Geometry: final body of the model. Coordinates: model frame, mm. A direction names the side the tool comes from. Give positions to 0.01 mm unless a question says otherwise; leave off trailing zeros. Loops run counter-clockwise (first coordinate to the right, second up) from the corner with the lowest first, then second, coordinate; pieces in that order, holes last.
from build123d import *

# Parameters (mm, degrees)
F1_DEPTH = 11.34999
F2_R     = 5.674985
F3_R     = 2.5
F4_DEPTH = 24.53132
F5_R     = 3.69316
F6_R     = 1.98374
F7_R     = 1.35255
F8_DEPTH = 1.70942


# Not quite as in the source:
# - a fillet or chamfer is up to 0.001 mm smaller than in the source, because OpenCascade refuses the exact size


with BuildPart() as f1:
    # F0 (on Top) → F1 (new body)
    with BuildSketch(Plane.XY):
        Polygon((-20.0249917, 0), (0, 0), (0, -21.11248), (-20.0249917, -21.11248), (-20.0249917, -22.8219), (1.70942, -22.8219), (1.70942, 1.70942), (-20.0249917, 1.70942), align=None)
    extrude(amount=F1_DEPTH)

    # F2 (radius 5.674995 in the source; OpenCascade refuses exactly that, so slightly less here)
    f2_edges = [f1.edges().sort_by_distance(p)[0] for p in [
        (-20.024992, -21.96719, 11.34999),
        (-20.024992, -21.96719, 0),
        (-20.024992, 0.85471, 11.34999),
        (-20.024992, 0.85471, 0),
    ]]
    fillet(f2_edges, radius=F2_R)

    # F3 (on face) → F4 (cut, through all)
    with BuildSketch(Plane.XZ.offset(22.8219)):
        with Locations((-14.3499967, 5.674995)):
            Circle(F3_R)
    extrude(amount=-F4_DEPTH, mode=Mode.SUBTRACT)

    # F5
    f5_edges = [f1.edges().sort_by_distance(p)[0] for p in [
        (1.70942, -22.8219, 5.674995),
        (1.70942, 1.70942, 5.674995),
    ]]
    fillet(f5_edges, radius=F5_R)

    # F6
    f6_edges = [f1.edges().sort_by_distance(p)[0] for p in [
        (0, -21.11248, 5.674995),
        (0, 0, 5.674995),
    ]]
    fillet(f6_edges, radius=F6_R)

    # F7 (on face) → F8 (cut, through all)
    with BuildSketch(Plane(origin=(0, 0, 0), x_dir=(0, -1, 0), z_dir=(-1, 0, 0))):
        with Locations((15.95374, 5.674995)):
            Circle(F7_R)
        with Locations((5.15874, 5.674995)):
            Circle(F7_R)
    extrude(amount=-F8_DEPTH, mode=Mode.SUBTRACT)


solid = f1.part
Item 1: Section query A-A on x = -8.5. Return loops of the section in (y, z).
Values follow:
outline: (-22.82, 0) - (-21.11, 0) - (-21.11, 11.35) - (-22.82, 11.35) - close; (0, 0) - (1.71, 0) - (1.71, 11.35) - (0, 11.35) - close
Item 2: Set-up query: faces 5 (the face through (-11, -21.112, 6)), 6 (the face through (1.709, -11, 6)). Return all of +Z, -Z, +X, -X, +Y, -Y with unobstructed straight access to the full face (end or side cutting, diameter ignored); none if empty.
Values follow:
face 5: +Z, -Z, -X
face 6: +Z, -Z, +X, +Y, -Y
Item 3: Section query D-D on y = -15.25. Return loops of the section in (x, z).
Values follow:
outline: (0, 0) - (1.71, 0) - (1.71, 4.52) - (0, 4.52) - close; (0, 6.83) - (1.71, 6.83) - (1.71, 11.35) - (0, 11.35) - close
Item 4: Pin query (flat end, axial travel): pin 1 (3.5 mm diameter, centred on y = -5.16, z = 5.67, fed in from +X); pin 2 (2 mm diameter, centred on y = -13.5, z = 5, fed in from -X). Return the tip coordinate at first contact, or that it passes through.
Values follow:
pin 1: stops at x = 1.71
pin 2: stops at x = 0
Item 5: Draft query along Z for faces 1 (the face through (-0.597, -0.566, 5.754)), 2 (the face through (-18.41, 0.84, 9.64)), 3 (the face through (-18.4, 0.8, 1.7)), 4 (the face through (-14.675, -21.979, 8.154)). Return one class per face: +Z half, -Z half, draft (parallel to the pull), parting line (faces both ways), or undercut.
Values follow:
face 1: draft
face 2: +Z half
face 3: -Z half
face 4: undercut
Item 6: Section query C-C on x = -13.25. Return loops of the section in (y, z).
Values follow:
outline: (-22.82, 0) - (-21.11, 0) - (-21.11, 3.43) - (-22.82, 3.43) - close; (-22.82, 7.92) - (-21.11, 7.92) - (-21.11, 11.35) - (-22.82, 11.35) - close; (0, 0) - (1.71, 0) - (1.71, 3.43) - (0, 3.43) - close; (0, 7.92) - (1.71, 7.92) - (1.71, 11.35) - (0, 11.35) - close
Item 7: Section query B-B on z = 6.5. Return loops of the section in (x, y), plus the area to 3 significant figures.
Values follow:
outline: (-19.96, -22.82) - (-16.71, -22.82) - (-16.71, -21.11) - (-19.96, -21.11) - close; (-19.96, 0) - (-16.71, 0) - (-16.71, 1.71) - (-19.96, 1.71) - close; (-11.99, -22.82) - (-1.98, -22.82) arc R3.69 ccw to (1.71, -19.13) - (1.71, -17.03) - (0, -17.03) - (0, -19.13) arc R1.98 cw to (-1.98, -21.11) - (-11.99, -21.11) - close; (-11.99, 0) - (-1.98, 0) arc R1.98 cw to (0, -1.98) - (0, -4.09) - (1.71, -4.09) - (1.71, -1.98) arc R3.69 ccw to (-1.98, 1.71) - (-11.99, 1.71) - close; (0, -14.88) - (1.71, -14.88) - (1.71, -6.23) - (0, -6.23) - close
area: 82.6 mm2
Item 8: Ray query, probe 1 along Y at (x, z) = (-12, 1); probe 2 along X at (y, z) = (-6, 7.75); probe 3 along Y at (x, z) = (-1.5, 4.5). Return the intervals inside material, ascending.
Values follow:
probe 1: y = -22.82 to -21.11, 0 to 1.71
probe 2: x = 0 to 1.71
probe 3: y = -22.79 to -21.05, -0.06 to 1.68
